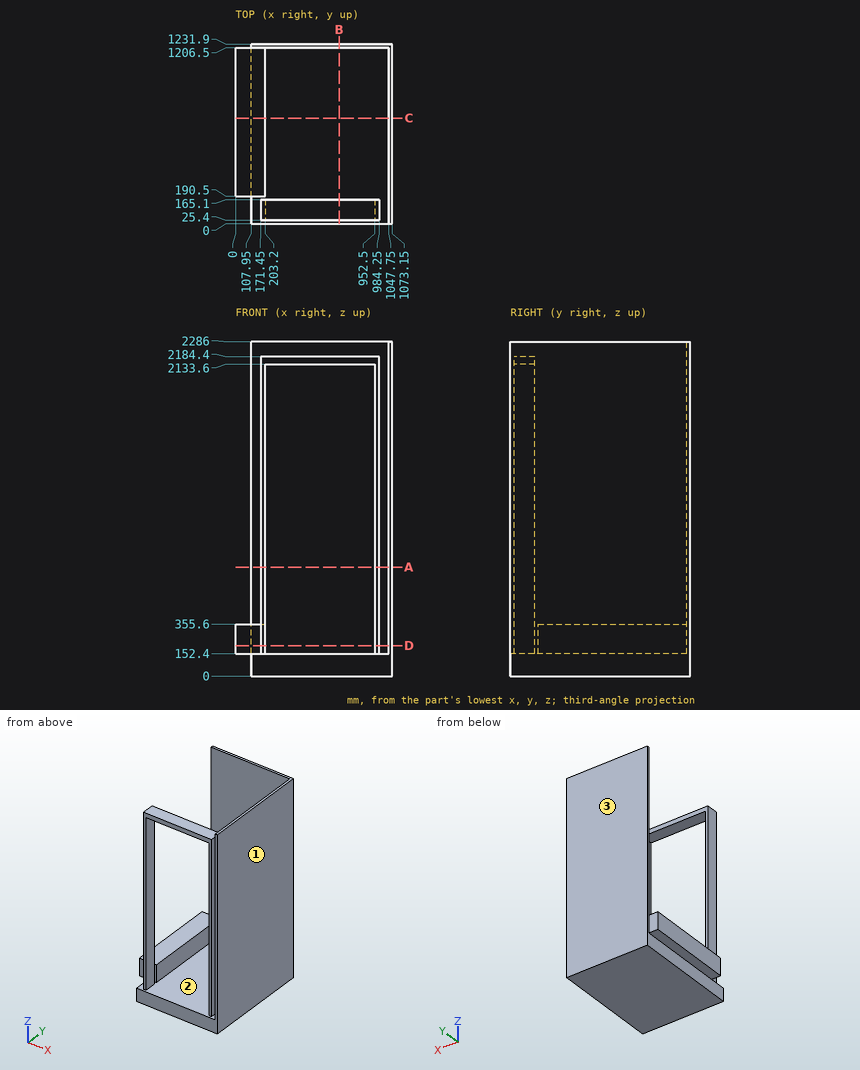
Answer from the drawing. Dimensions are ordinates in mm from the lowest x, y and z of the part. Round coordinates to 2 decimals unless told otherwise and drop trailing zeros. Write each loop counter-clockwise with the first axis right and the second up, starting at its lowest first coordinate (ties: lowest second). Pieces come first, ordered by that corner, then holes.
1. The part is cut by section C-C, the plane y = 725. Determine the outline of the cut face in (x, z), then the cut area to 3 significant figures.
2. The part is cut by section B-B, the plane x = 708.5. Determine the outline of the cut face in (y, z).
3. The part is cut by section D-D, the plane z = 208.5. Determine the outline of the cut face in (x, y), then the cut area to 3 significant figures.
4. Determine the mould class of the marked faces 1, 2 and 3 for opening direction X: pulls with the +X half, pulls with the -X half, needs draft (parallel to the pull), parting line crosses it, or undercut.
5. Given pin 1 Ø10 at (x, y) = (832, 286) entering from +Z; pin 2 Ø3 at (x, z) = (473, 1636) entering from -Y; pin 3 Ø3 at (y, z) = (183.5, 345) entering from -X, each flat-ended and moving along its own axis, determine where each tip first touches the part or whether it passes through.
6. The part is cut by section A-A, the plane z = 746. Determine the outline of the cut face in (x, y), then the cut area to 3 significant figures.
7. Straight lines are drawn through the part: L1, parallel to X at y = 110, z = 1168; L2, parallel to Z at x = 542, y = 102; L3, parallel to X at y = 535, z = 531.5. For each, find the intervals that lie inside material, in ascending order.
Values:
1. outline: (0, 152.4) - (107.95, 152.4) - (107.95, 0) - (1073.15, 0) - (1073.15, 2286) - (1047.75, 2286) - (1047.75, 152.4) - (203.2, 152.4) - (203.2, 355.6) - (0, 355.6) - close
1. area: 243,000 mm2
2. outline: (0, 0) - (1231.9, 0) - (1231.9, 2286) - (1206.5, 2286) - (1206.5, 152.4) - (0, 152.4) - close; (25.4, 2133.6) - (165.1, 2133.6) - (165.1, 2184.4) - (25.4, 2184.4) - close
3. outline: (0, 190.5) - (203.2, 190.5) - (203.2, 1206.5) - (1047.75, 1206.5) - (1047.75, 0) - (1073.15, 0) - (1073.15, 1231.9) - (107.95, 1231.9) - (107.95, 1206.5) - (0, 1206.5) - close; (171.45, 25.4) - (203.2, 25.4) - (203.2, 165.1) - (171.45, 165.1) - close; (952.5, 25.4) - (984.25, 25.4) - (984.25, 165.1) - (952.5, 165.1) - close
3. area: 270,000 mm2
4. face 1: pulls with the +X half
4. face 2: undercut
4. face 3: needs draft
5. pin 1: stops at z = 152.4
5. pin 2: stops at y = 1206.5
5. pin 3: stops at x = 1047.75
6. outline: (107.95, 1206.5) - (1047.75, 1206.5) - (1047.75, 0) - (1073.15, 0) - (1073.15, 1231.9) - (107.95, 1231.9) - close; (171.45, 25.4) - (203.2, 25.4) - (203.2, 165.1) - (171.45, 165.1) - close; (952.5, 25.4) - (984.25, 25.4) - (984.25, 165.1) - (952.5, 165.1) - close
6. area: 64,000 mm2
7. L1: x = 171.45 to 203.2, 952.5 to 984.25, 1047.75 to 1073.15
7. L2: z = 0 to 152.4, 2133.6 to 2184.4
7. L3: x = 1047.75 to 1073.15
